```python
from build123d import *

# Parameters (mm, degrees)
BOSS_EXTRUDE1_DEPTH     = 1.5875
SKETCH2_R               = 2.4892
CUT_EXTRUDE1_DEPTH      = 1
CUT_EXTRUDE1_DEPTH_BACK = 2.5875
FILLET1_R               = 3.175


with BuildPart() as part:
    # Sketch1 → Boss-Extrude1 (new body)
    with BuildSketch(Plane(origin=(0, 0, 0), x_dir=(1, 0, 0), z_dir=(0, 1, 0))):
        Polygon((12.7, 12.7), (63.5, 12.7), (63.5, -12.7), (-63.5, -12.7), (-63.5, 12.7), (-12.7, 12.7), (-12.7, 88.9), (12.7, 88.9), align=None)
    extrude(amount=BOSS_EXTRUDE1_DEPTH)

    # Sketch2 → Cut-Extrude1 (cut, two sides)
    with BuildSketch(Plane(origin=(0, 1.5875, 0), x_dir=(1, 0, 0), z_dir=(0, 1, 0))) as cut_extrude1_sk:
        Circle(SKETCH2_R)
        with Locations((0, 25.4)):
            Circle(SKETCH2_R)
        with Locations((0, 50.8)):
            Circle(SKETCH2_R)
        with Locations((0, 76.2)):
            Circle(SKETCH2_R)
        with Locations((-25.4, 0)):
            Circle(SKETCH2_R)
        with Locations((-50.8, 0)):
            Circle(SKETCH2_R)
        with Locations((25.4, 0)):
            Circle(SKETCH2_R)
        with Locations((50.8, 0)):
            Circle(SKETCH2_R)
    extrude(amount=CUT_EXTRUDE1_DEPTH, mode=Mode.SUBTRACT)
    extrude(cut_extrude1_sk.sketch, amount=-CUT_EXTRUDE1_DEPTH_BACK, mode=Mode.SUBTRACT)

    # Fillet1
    fillet1_edges = [part.edges().sort_by_distance(p)[0] for p in [
        (63.5, 0.79375, 12.7),
        (-63.5, 0.79375, 12.7),
        (-63.5, 0.79375, -12.7),
        (-12.7, 0.79375, -12.7),
        (-12.7, 0.79375, -88.9),
        (12.7, 0.79375, -88.9),
        (12.7, 0.79375, -12.7),
        (63.5, 0.79375, -12.7),
    ]]
    fillet(fillet1_edges, radius=FILLET1_R)


solid = part.part
```
Build history of the part. All positions in model axes, mm. Round coordinates to 2 decimals unless told otherwise and drop trailing zeros. Loops run counter-clockwise (first coordinate to the right, second up) from the corner with the lowest first, then second, coordinate; pieces in that order, holes last. Notation, with made-up numbers: M -11,10.5 L 44,10.5 A30 ccw 44,33.5 Z; hole C -0.5,-21.75 d10. An arc over 180 degrees is marked long. Answer as CSV lines item,"result".
1. Flat gauge pins, fed straight in: P1, Ø5.5, axis at x = 0, z = -50.8, coming from the -Y side; P2, Ø0.5, axis at x = -41.5, y = 0.5, coming from the -Z side; P3, Ø0.5, axis at y = 0.5, z = -51.5, coming from the +X side; P4, Ø4, axis at x = 0, z = -25.4, coming from the +Y side. Where does each tip first touch, or does it go through?
Resolved:
P1,"stops at y = 0"
P2,"stops at z = -12.7"
P3,"stops at x = 12.7"
P4,"passes through"
2. Wall check: probe 1 along X at (y, z) = (0.4, 0); probe 2 along Z at (x, y) = (0, 0.55); probe 3 along X at (y, z) = (0.8, -76). Give the ranges that are in metal, low to high. Write a range as [from, to].
Resolved:
probe 1,"x = [-63.5, -53.29], [-48.31, -27.89], [-22.91, -2.49], [2.49, 22.91], [27.89, 48.31], [53.29, 63.5]"
probe 2,"z = [-88.9, -78.69], [-73.71, -53.29], [-48.31, -27.89], [-22.91, -2.49], [2.49, 12.7]"
probe 3,"x = [-12.7, -2.48], [2.48, 12.7]"
3. Cut at D-D on y = 0.45. Count the separate pieces of the cut face and the enclosed holes in it, then the cut area to 3 significant figures.
Resolved:
separate pieces,"1"
enclosed holes,"8"
area,"5,000 mm²"
4. Two-plate mould, pull along Z, no slides. Class faces 1 (the cylindrical face through (62.59, 0.8, 11.75)), 2 (the cylindrical face through (-11.75, 0.8, -87.99)), 3 (the cylindrical face through (53.1, 0.8, 0.95)): released by +Z, released by -Z, zero draft, split by the parting line, or undercut.
Resolved:
face 1,"released by +Z"
face 2,"released by -Z"
face 3,"undercut"
5. Cut at A-A on z = 0. Write the cut outline in (x, y).
Resolved:
outline,"M -63.5,0 L -53.29,0 L -53.29,1.59 L -63.5,1.59 Z; M -48.31,0 L -27.89,0 L -27.89,1.59 L -48.31,1.59 Z; M -22.91,0 L -2.49,0 L -2.49,1.59 L -22.91,1.59 Z; M 2.49,0 L 22.91,0 L 22.91,1.59 L 2.49,1.59 Z; M 27.89,0 L 48.31,0 L 48.31,1.59 L 27.89,1.59 Z; M 53.29,0 L 63.5,0 L 63.5,1.59 L 53.29,1.59 Z"
6. Cut at B-B on x = 25.4. Write the cut outline in (y, z), then the cut area to 3 significant figures.
Resolved:
outline,"M 0,-12.7 L 1.59,-12.7 L 1.59,-2.49 L 0,-2.49 Z; M 0,2.49 L 1.59,2.49 L 1.59,12.7 L 0,12.7 Z"
area,"32.4 mm²"
7. Cut at C-C on z = -50.8. Write the cut outline in (x, y), then the cut area to 3 significant figures.
Resolved:
outline,"M -12.7,0 L -2.49,0 L -2.49,1.59 L -12.7,1.59 Z; M 2.49,0 L 12.7,0 L 12.7,1.59 L 2.49,1.59 Z"
area,"32.4 mm²"
